Geometry: final body of the model. Coordinates: model frame, mm. Coordinates: 2 decimals unless noted, no trailing zeros. Loops run counter-clockwise (first coordinate to the right, second up) from the corner with the lowest first, then second, coordinate; pieces in that order, holes last. Notation, with made-up numbers: (8.5, 84) - (24.5, 84) arc R13 ccw to (24.5, 95) - close; hole circle Ø4 at (19, 6). An arc over 180 degrees is marked (long way). Answer in a Markdown table with one row per item.
from build123d import *

# Parameters (mm, degrees)
SKETCH1_W           = 101
SKETCH1_H           = 8
SKETCH1_W_2         = 99
SKETCH1_H_2         = 6
BOSS_EXTRUDE1_DEPTH = 10
SKETCH2_R           = 1.2
BOSS_EXTRUDE2_DEPTH = 2
SKETCH3_W           = 103
SKETCH3_H           = 10
SKETCH3_W_2         = 101
SKETCH3_H_2         = 8
BOSS_EXTRUDE3_DEPTH = 6
FILLET4_R           = 1
FILLET5_R           = 1
FILLET6_R           = 1
FILLET7_R           = 1
FILLET8_R           = 0.5
FILLET9_R           = 0.5
CUT_EXTRUDE1_DEPTH  = 2
CUT_EXTRUDE2_DEPTH  = 0.5


# Some blends are built 0.0001 mm under size
with BuildPart() as part:
    # Sketch1 → Boss-Extrude1 (new body)
    with BuildSketch(Plane(origin=(0, 0, 0), x_dir=(1, 0, 0), z_dir=(0, 1, 0))):
        Rectangle(SKETCH1_W, SKETCH1_H)
        Rectangle(SKETCH1_W_2, SKETCH1_H_2, mode=Mode.SUBTRACT)
    extrude(amount=BOSS_EXTRUDE1_DEPTH)

    # Sketch2 → Boss-Extrude2 (add)
    # profile 1 of 3: a face of its own
    with BuildSketch(Plane.XZ):
        with BuildLine():
            Line((48, 4), (50.5, 4))
            Line((50.5, 4), (50.5, 13))
            ThreePointArc((50.5, 13), (46.232233047, 14.767766953), (48, 10.5))
            Line((48, 10.5), (48, 4))
        make_face()
        with Locations(Location((48, 13, 0), (0, 0, 270))):
            Circle(SKETCH2_R, mode=Mode.SUBTRACT)
    # profile 2 of 3: a face of its own
    with BuildSketch(Plane.XZ):
        with BuildLine():
            Line((48, -4), (50.5, -4))
            Line((50.5, -4), (50.5, -11))
            ThreePointArc((50.5, -11), (46.232233047, -12.767766953), (48, -8.5))
            Line((48, -8.5), (48, -4))
        make_face()
        with Locations(Location((48, -11, 0), (0, 0, 270))):
            Circle(SKETCH2_R, mode=Mode.SUBTRACT)
    # profile 3 of 3: a face of its own
    with BuildSketch(Plane.XZ):
        with BuildLine():
            Line((-66.4, 15), (-48.835058433, 15))
            Line((-48.835058433, 15), (-48.835058433, 4))
            Line((-48.835058433, 4), (-50.5, 4))
            Line((-50.5, 4), (-50.5, -4))
            Line((-50.5, -4), (-51.901659191, -4))
            Line((-51.901659191, -4), (-51.901659191, 11))
            Line((-51.901659191, 11), (-66.4, 11))
            ThreePointArc((-66.4, 11), (-68.4, 13), (-66.4, 15))
        make_face()
        with Locations(Location((-66.4, 13, 0), (0, 0, 270))):
            Circle(SKETCH2_R, mode=Mode.SUBTRACT)
    extrude(amount=-BOSS_EXTRUDE2_DEPTH)

    # Sketch3 → Boss-Extrude3 (add)
    with BuildSketch(Plane(origin=(0, 10, 0), x_dir=(1, 0, 0), z_dir=(0, 1, 0))):
        Rectangle(SKETCH3_W, SKETCH3_H)
        Rectangle(SKETCH3_W_2, SKETCH3_H_2, mode=Mode.SUBTRACT)
    extrude(amount=-BOSS_EXTRUDE3_DEPTH)

    # Fillet4
    fillet4_edges = [part.edges().sort_by_distance(p)[0] for p in [
        (0, 4, -4),
    ]]
    fillet(fillet4_edges, radius=FILLET4_R - 0.0001)  # a hair under: the kernel refuses the full size

    # Fillet5
    fillet5_edges = [part.edges().sort_by_distance(p)[0] for p in [
        (0, 4, 4),
    ]]
    fillet(fillet5_edges, radius=FILLET5_R - 0.0001)  # a hair under: the kernel refuses the full size

    # Fillet6
    fillet6_edges = [part.edges().sort_by_distance(p)[0] for p in [
        (50.5, 4, 0),
    ]]
    fillet(fillet6_edges, radius=FILLET6_R - 0.0001)  # a hair under: the kernel refuses the full size

    # Fillet7
    fillet7_edges = [part.edges().sort_by_distance(p)[0] for p in [
        (-50.5, 4, 0),
    ]]
    fillet(fillet7_edges, radius=FILLET7_R - 0.0001)  # a hair under: the kernel refuses the full size

    # Fillet8
    fillet8_edges = [part.edges().sort_by_distance(p)[0] for p in [
        (-51.901659191, 1, 11),
        (-48.835058433, 1, 15),
    ]]
    fillet(fillet8_edges, radius=FILLET8_R)

    # Fillet9
    # the kernel refuses this fillet: 0.5 mm, written as the material it takes off along each edge
    with BuildSketch(Plane(origin=(51.5, 11.25, -5), x_dir=(-1, 0, 0), z_dir=(0, -1, 0))) as fillet9_piece_1:
        with BuildLine():
            CenterArc((FILLET9_R, -FILLET9_R), FILLET9_R, 90, 90)
            Line((0, -FILLET9_R), (0, 0))
            Line((0, 0), (FILLET9_R, 0))
        make_face()
    extrude(amount=8.5, mode=Mode.SUBTRACT)
    with BuildSketch(Plane(origin=(51.5, 11.25, 5), x_dir=(-1, 0, 0), z_dir=(0, -1, 0)), Plane(origin=(-51.5, 11.25, 5), x_dir=(0, 0, -1), z_dir=(0, -1, 0)), Plane(origin=(-51.5, 11.25, -5), x_dir=(1, 0, 0), z_dir=(0, -1, 0))) as fillet9_piece_2:
        with BuildLine():
            CenterArc((FILLET9_R, FILLET9_R), FILLET9_R, 180, 90)
            Line((0, FILLET9_R), (0, 0))
            Line((0, 0), (FILLET9_R, 0))
        make_face()
    extrude(amount=8.5, mode=Mode.SUBTRACT)

    # Sketch4 → Cut-Extrude1 (cut)
    with BuildSketch(Plane(origin=(0, 10, 0), x_dir=(1, 0, 0), z_dir=(0, 1, 0))):
        with BuildLine():
            Line((51.5, -4.5), (51.5, 4.5))
            ThreePointArc((51.5, 4.5), (51.353553391, 4.853553391), (51, 5))
            Line((51, 5), (-51, 5))
            ThreePointArc((-51, 5), (-51.353553391, 4.853553391), (-51.5, 4.5))
            Line((-51.5, 4.5), (-51.5, -4.5))
            ThreePointArc((-51.5, -4.5), (-51.353553391, -4.853553391), (-51, -5))
            Line((-51, -5), (51, -5))
            ThreePointArc((51, -5), (51.353553391, -4.853553391), (51.5, -4.5))
        make_face()
    extrude(amount=-CUT_EXTRUDE1_DEPTH, mode=Mode.SUBTRACT)

    # Sketch5 → Cut-Extrude2 (cut)
    # profile 1 of 2: a face of its own
    with BuildSketch(Plane.XY.offset(4)):
        Polygon((0.128205128, 2.5), (0.368589744, 2.5), (1.201923077, 0.529847756), (2.03525641, 2.5), (2.275641026, 2.5), (1.217948718, 0), (1.185897436, 0), align=None)
    # profile 2 of 2: a face of its own
    with BuildSketch(Plane.XY.offset(4)):
        Polygon((3.864683494, 2.564102564), (3.91025641, 2.564102564), (3.91025641, 0.833333333), (4.198717949, 0.833333333), (4.198717949, 0.576923077), (3.91025641, 0.576923077), (3.91025641, 0), (3.685897436, 0), (3.685897436, 0.576923077), (2.5, 0.576923077), align=None)
        Polygon((3.685897436, 0.833333333), (3.685897436, 1.919070513), (2.940705128, 0.833333333), align=None, mode=Mode.SUBTRACT)
    extrude(amount=-CUT_EXTRUDE2_DEPTH, mode=Mode.SUBTRACT)


solid = part.part
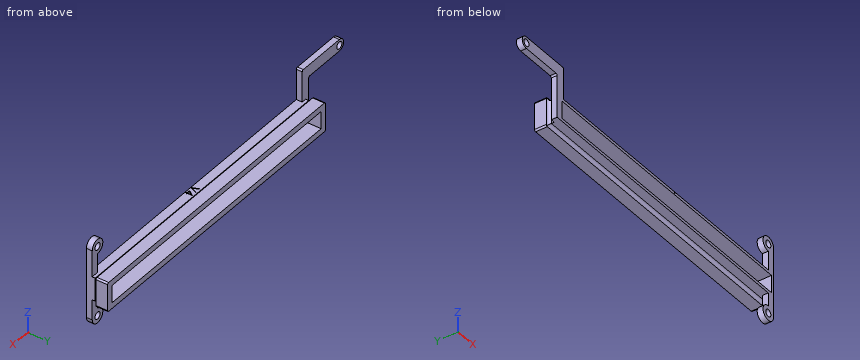
(1) Ray query, probe 1 along X at (y, z) = (0.5, 13); probe 2 along Z at (x, y) = (-12.5, 6.25); probe 3 along X at (y, z) = (0.9, -11). Return the intervals inside material, ascending.
Verdict:
| item | result |
|---|---|
| probe 1 | x = -68.4 to -67.6, -65.2 to -48.84, 45.5 to 46.8, 49.2 to 50.5 |
| probe 2 | z = -5 to -3, 3 to 5 |
| probe 3 | x = 45.5 to 46.8, 49.2 to 50.5 |
(2) Cut plane B-B on z = 6.25. Output: boundary loops of the cut face in (x, y).
Verdict:
| item | result |
|---|---|
| outline | (-51.9, 0) - (-48.84, 0) - (-48.84, 2) - (-51.9, 2) - close; (48, 0) - (50.5, 0) - (50.5, 2) - (48, 2) - close |
(3) Cut plane C-C on y = 5.25. Output: boundary loops of the cut face in (x, z), then the cut area to 3 significant figures.
Verdict:
| item | result |
|---|---|
| outline | (-51.5, -4.5) arc R0.5 ccw to (-51, -5) - (51, -5) arc R0.5 ccw to (51.5, -4.5) - (51.5, 4.5) arc R0.5 ccw to (51, 5) - (-51, 5) arc R0.5 ccw to (-51.5, 4.5) - close; hole (-49.5, -3) - (49.5, -3) - (49.5, 3) - (-49.5, 3) - close |
| area | 436 mm² |
(4) First-contact query: pin 1 Ø1.5 at (x, y) = (-48, 7) entering from +Z; pin 2 Ø1.9 at (x, y) = (3, 1.5) entering from +Z; pin 3 Ø3 at (y, z) = (2, -1.5) entering from -X. Flat tips, straight axial feed; report the tip coordinate or a pass-through.
Verdict:
| item | result |
|---|---|
| pin 1 | stops at z = 5 |
| pin 2 | stops at z = 4 |
| pin 3 | stops at x = -51.9 |
